Design review of the part built by this model. Coordinates are the model's own, in mm. A direction names the side the tool comes from. Coordinates: 2 decimals unless noted, no trailing zeros. Order: outer loops, then holes, each group sorted by start corner. A loop starts at its lowest first (then second) coordinate and runs counter-clockwise, first axis right, second up. Notation, with made-up numbers: (59, 78.25) -> (89, 78.25) arc R20 cw to (89, 94.25) -> close; hole circle Ø9 at (81.5, 22.25). An arc over 180 degrees is marked (long way). Use a Markdown table: item, result. Add a question column.
Q1. Wall thickness on probe 1 along Y at (x, z) = (21, 3.55); probe 2 along Z at (x, y) = (-23, -5.5); probe 3 along X at (y, z) = (-4.5, 4.05): over which ranges is each line inside the solid? List them lowest first.
Q2. Insertion check: pin 1 (1.5 mm diameter, centred on x = 3, y = 8.5, fed in from +Z); pin 2 (2 mm diameter, centred on x = -2.5, z = 2.5, fed in from -Y); pin 3 (1.7 mm diameter, centred on x = -7, z = 4, fed in from +Y). Each pin has a flat end and moves straight along its axis. Give the tip position at first contact, or say it passes through.
Q3. Add section D-D (y = -8.25). State the section outline as (x, z) points.
Q4. Machinability: for faces 4 (the face through (-23.65, 8.68, 0.81)), 5 (the face through (1, 9, 1.6)), 6 (the face through (-23.67, -8.64, 0.79)), 7 (the face through (-1, 0, 1.6)), which of the approach directions +Z, -Z, +X, -X, +Y, -Y give a long, thin tool a straight path to every point of the face, cutting with its end or side? Answer none if there is none.
Q5. Add section A-A (z = 3.25). State the section outline as (x, y) points.
Q6. Add section B-B (y = 2.25). State the section outline as (x, z) points, then the cut area to 3 significant figures.
Q7. Add section C-C (x = -19). State the section outline as (y, z) points, then the cut area to 3 significant figures.
Q8. The part is to be moulded in two halves that separate along Y. For faces 1 (the face through (0.819, 9.875, 0.301)), 2 (the face through (23.9, 0, 4)), 3 (the face through (1, -9, 1.6)), say which applies: pulls with the +Y half, pulls with the -Y half, needs draft (parallel to the pull), parting line crosses it, or undercut.
from build123d import *

# Parameters (mm, degrees)
F0_W        = 50.8
F0_H        = 20.32
F1_DEPTH    = 1.6
F2_W        = 1.5
F2_H        = 11.32
F3_DEPTH    = 4
F4_R        = 1
F5_T1_DEPTH = 9.5320747894
F5_T3_DEPTH = 9.5320747894


# Not quite as in the source:
# - a fillet or chamfer that OpenCascade refuses, or shapes differently, is made with other operations: its cross-section is extruded or revolved along the edge and cut away or added


with BuildPart() as f1:
    # F0 (on Top) → F1 (new body)
    with BuildSketch(Plane.XY):
        Rectangle(F0_W, F0_H)
    extrude(amount=F1_DEPTH)

    # F2 (on face) → F3 (join)
    with BuildSketch(Plane.XY.offset(1.6)):
        Polygon((25.4, 7.16), (-25.4, 7.16), (-25.4, 5.66), (23.9, 5.66), (25.4, 5.66), align=None)
        with Locations((24.65, 0)):
            Rectangle(F2_W, F2_H)
        Polygon((25.4, -7.16), (25.4, -5.66), (23.9, -5.66), (-25.4, -5.66), (-25.4, -7.16), align=None)
    extrude(amount=F3_DEPTH)

    # F4
    f4_edges = [f1.edges().sort_by_distance(p)[0] for p in [
        (0, -10.16, 0),
        (0, 10.16, 0),
    ]]
    fillet(f4_edges, radius=F4_R)

    # F5: chamfer of 2.54 on 2 edges, made by hand

    # F5_s2 → F5_t1 (cut)
    with BuildSketch(Plane.XZ.offset(-16.6920747894)):
        Polygon((-22.86, 1.6), (-25.4, -0.94), (-25.4, 1.6), align=None)
    extrude(amount=F5_T1_DEPTH, mode=Mode.SUBTRACT)

    # F5_s4 → F5_t3 (cut)
    with BuildSketch(Plane.XZ.offset(7.16)):
        Polygon((-25.4, -0.94), (-22.86, 1.6), (-25.4, 1.6), align=None)
    extrude(amount=F5_T3_DEPTH, mode=Mode.SUBTRACT)


solid = f1.part
Established:
| question | item | result |
|---|---|---|
| 1 | probe 1 | -7.16 to -5.66, 5.66 to 7.16 |
| 1 | probe 2 | 0 to 1.6 |
| 1 | probe 3 | 23.9 to 25.4 |
| 2 | pin 1 | z = 1.6 |
| 2 | pin 2 | y = -10.16 |
| 2 | pin 3 | y = 7.16 |
| 3 | outline | (-24.46, 0) -> (25.4, 0) -> (25.4, 1.6) -> (-22.86, 1.6) -> close |
| 4 | face 4 | +Z, -X, +Y |
| 4 | face 5 | +Z, +X, -X, +Y |
| 4 | face 6 | +Z, -X, -Y |
| 4 | face 7 | +Z, -X |
| 5 | outline | (-25.4, -7.16) -> (25.4, -7.16) -> (25.4, 7.16) -> (-25.4, 7.16) -> (-25.4, 5.66) -> (23.9, 5.66) -> (23.9, -5.66) -> (-25.4, -5.66) -> close |
| 6 | outline | (-25.4, 0) -> (25.4, 0) -> (25.4, 5.6) -> (23.9, 5.6) -> (23.9, 1.6) -> (-25.4, 1.6) -> close |
| 6 | area | 87.3 mm^2 |
| 7 | outline | (-10.16, 1) arc R1 ccw to (-9.16, 0) -> (9.16, 0) arc R1 ccw to (10.16, 1) -> (10.16, 1.6) -> (7.16, 1.6) -> (7.16, 5.6) -> (5.66, 5.6) -> (5.66, 1.6) -> (-5.66, 1.6) -> (-5.66, 5.6) -> (-7.16, 5.6) -> (-7.16, 1.6) -> (-10.16, 1.6) -> close |
| 7 | area | 44.1 mm^2 |
| 8 | face 1 | pulls with the +Y half |
| 8 | face 2 | undercut |
| 8 | face 3 | needs draft |
